Build history of the part. All positions in model axes, mm. A direction names the side the tool comes from. Give positions to 0.01 mm unless a question says otherwise; leave off trailing zeros. Write each loop counter-clockwise with the first axis right and the second up, starting at its lowest first coordinate (ties: lowest second). Pieces come first, ordered by that corner, then holes.
from build123d import *

# Parameters (mm, degrees)
ESQUISSE1_R        = 150
BOSS_EXTRU_1_DEPTH = 250
ESQUISSE2_R        = 70
BOSS_EXTRU_2_DEPTH = 10
ESQUISSE3_W        = 370
ESQUISSE3_H        = 241.309251742
BOSS_EXTRU_3_DEPTH = 40
ESQUISSE4_W        = 40
ESQUISSE4_H        = 241.309251742
BOSS_EXTRU_4_DEPTH = 370
ESQUISSE5_R        = 70
BOSS_EXTRU_5_DEPTH = 10


with BuildPart() as part:
    # Esquisse1 → Boss.-Extru.1 (new body)
    with BuildSketch(Plane.XY):
        Circle(ESQUISSE1_R)
    extrude(amount=BOSS_EXTRU_1_DEPTH)

    # Esquisse2 → Boss.-Extru.2 (add)
    with BuildSketch(Plane(origin=(0, 0, 0), x_dir=(-1, 0, 0), z_dir=(0, 0, -1))):
        Circle(ESQUISSE2_R)
    extrude(amount=BOSS_EXTRU_2_DEPTH)

    # Esquisse3 → Boss.-Extru.3 (add)
    with BuildSketch(Plane.XY.offset(250)):
        Rectangle(ESQUISSE3_W, ESQUISSE3_H)
    extrude(amount=BOSS_EXTRU_3_DEPTH)

    # Esquisse4 → Boss.-Extru.4 (add)
    with BuildSketch(Plane.XY.offset(290)):
        with Locations((-165, 0)):
            Rectangle(ESQUISSE4_W, ESQUISSE4_H)
        with Locations((165, 0)):
            Rectangle(ESQUISSE4_W, ESQUISSE4_H)
    extrude(amount=BOSS_EXTRU_4_DEPTH)

    # Esquisse5 → Boss.-Extru.5 (add)
    with BuildSketch(Plane.ZY.offset(-145)):
        with Locations(Location((560, -0.654625871, 0), (0, 0, 180))):
            Circle(ESQUISSE5_R)
    extrude(amount=BOSS_EXTRU_5_DEPTH)


solid = part.part
(1) 3-axis set-ups, long thin cutter, end or side, ignore diameter. For faces 5 (the face through (158, 2, 250)), 6 (the face through (55.55, -42.594, -4.93)), 7 (the face through (-15, 120.655, 287)): which of +Z, -Z, +X, -X, +Y, -Y reach the whole face in a straight line?
(2) Mould opens along X. For faces 1 (the face through (-1, 132, 250)), 2 (the face through (-19.527, 148.724, 123.25)), 3 (the face through (185, -2, 452)), 4 (the face through (140.07, 26.16, 495.34)) say: +X half, -X half, draft (parallel to the pull), parting line (faces both ways), or undercut.
(3) Saw through at C-C, the plane y = -109. List the corners of the cut face in (x, z).
(4) Saw through at B-B, the plane x = 0. List the corners of the cut face in (y, z), plus the area to 3 significant figures.
(5) Saw through at A-A, the plane z = 560. List the corners of the cut face in (x, y).
(6) Saw through at D-D, the plane z = 480. List the corners of the cut face in (x, y).
(7) Probe line 1 (X direction, y = -74, z = 587); line 2 (X direction, y = 49, z = 516); line 3 (Z direction, x = 110, y = 54.5). List the from-to ranges inside material, lowest first.
(8) Drop flat-ended pins along their axis: pin 1 (9 mm diameter, centred on x = 12, y = -135.5, fed in from +Z); pin 2 (2 mm diameter, centred on x = -80, y = -63.5, fed in from -Z); pin 3 (1 mm diameter, centred on x = -35.5, y = 112, fed in from +Z). Give the stop position or say it passes through.
Computed values:
1. face 5: -Z, +X
1. face 6: -Z
1. face 7: +Z, +X, -X, +Y
2. face 1: draft
2. face 2: parting line
2. face 3: +X half
2. face 4: undercut
3. outline: (-185, 250) - (-103.05, 250) - (-103.05, 0) - (103.05, 0) - (103.05, 250) - (185, 250) - (185, 660) - (145, 660) - (145, 290) - (-145, 290) - (-145, 660) - (-185, 660) - close
4. outline: (-150, 0) - (-70, 0) - (-70, -10) - (70, -10) - (70, 0) - (150, 0) - (150, 250) - (120.65, 250) - (120.65, 290) - (-120.65, 290) - (-120.65, 250) - (-150, 250) - close
4. area: 86,100 mm2
5. outline: (-185, -120.65) - (-145, -120.65) - (-145, 120.65) - (-185, 120.65) - close; (135, -70.65) - (145, -70.65) - (145, -120.65) - (185, -120.65) - (185, 120.65) - (145, 120.65) - (145, 69.35) - (135, 69.35) - close
6. outline: (-185, -120.65) - (-145, -120.65) - (-145, 120.65) - (-185, 120.65) - close; (145, -120.65) - (185, -120.65) - (185, 120.65) - (145, 120.65) - close
7. line 1: x = -185 to -145, 145 to 185
7. line 2: x = -185 to -145, 135 to 185
7. line 3: z = 0 to 290
8. pin 1: stops at z = 250
8. pin 2: stops at z = 0
8. pin 3: stops at z = 290
